Input: dimensioned drawing with shaded views. Units: mm. Origin: part minimum x, y, z. A direction names the side the tool comes from. Round coordinates to 2 decimals unless told otherwise and drop trailing zeros. Loops run counter-clockwise (first coordinate to the right, second up) from the corner with the lowest first, then second, coordinate; pieces in that order, holes last. Notation, with made-up numbers: M -15,22.25 L 42,22.25 A35 ccw 42,54.25 Z; hole C -26,21.5 d4. An arc over 180 degrees is marked long. Use one line per item in the form item = value. Start each with the question number.
Q1. Ray query, line 1 along Z through (x, y) = (12, 0.8); line 2 along X through (y, z) = (3.25, 20); line 3 along Z through (x, y) = (60.8, 21.95). Return the intervals inside material, ascending.
Q2. Section query A-A, the plane x = 60.8. Output: boundary loops of the cut face in (y, z).
Q3. Access query for the marked faces 1, 2 and 3. Directions: +Z, -Z, +X, -X, +Y, -Y. A direction counts if a zero-diameter tool reaches every point of the face in a straight line with its end or side. Return the directions, or none.
Q4. First-contact query: P1, Ø4, axis at x = 12, z = 37.5, coming from the -Y side; P2, Ø2, axis at y = 8.5, z = 15.5, coming from the -X side; P3, Ø5, axis at x = 12, z = 17.5, coming from the +Y side; P4, Ø16, axis at x = 60.8, z = 27.5, coming from the -Y side. Flat tips, straight axial feed; report the tip coordinate or a pass-through.
Q5. Section query C-C, the plane x = 12. Output: boundary loops of the cut face in (y, z).
Q6. Section query D-D, the plane z = 37.5. Output: boundary loops of the cut face in (x, y), and give its area (3 significant figures).
Q7. Section query B-B, the plane z = 27.5. Output: boundary loops of the cut face in (x, y), and give its area (3 significant figures).
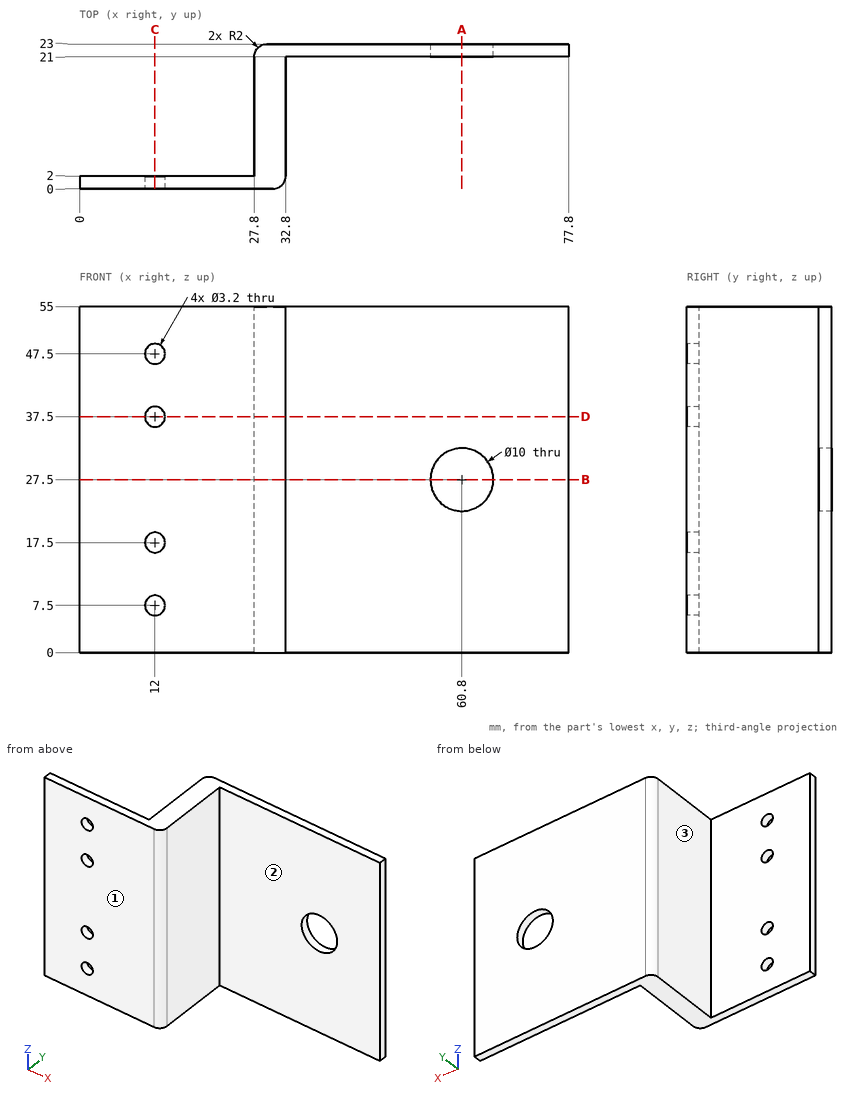
Results found:
q1.line_1 = 0 to 5.9, 9.1 to 15.9, 19.1 to 35.9, 39.1 to 45.9, 49.1 to 55
q1.line_2 = 27.8 to 32.8
q1.line_3 = 0 to 22.5, 32.5 to 55
q2.outline = M 21,0 L 23,0 L 23,22.5 L 21,22.5 Z; M 21,32.5 L 23,32.5 L 23,55 L 21,55 Z
q3.face_1 = +Z, -Z, +X, -X, -Y
q3.face_2 = +Z, -Z, +X, -Y
q3.face_3 = +Z, -Z, -X, +Y
q4.P1 = 0
q4.P2 = 27.8
q4.P3 = 2
q4.P4 = 21
q5.outline = M 0,0 L 2,0 L 2,5.9 L 0,5.9 Z; M 0,9.1 L 2,9.1 L 2,15.9 L 0,15.9 Z; M 0,19.1 L 2,19.1 L 2,35.9 L 0,35.9 Z; M 0,39.1 L 2,39.1 L 2,45.9 L 0,45.9 Z; M 0,49.1 L 2,49.1 L 2,55 L 0,55 Z
q6.outline = M 0,0 L 10.4,0 L 10.4,2 L 0,2 Z; M 13.6,0 L 30.8,0 A2 ccw 32.8,2 L 32.8,21 L 77.8,21 L 77.8,23 L 29.8,23 A2 ccw 27.8,21 L 27.8,2 L 13.6,2 Z
q6.area = 252 mm²
q7.outline = M 0,0 L 30.8,0 A2 ccw 32.8,2 L 32.8,21 L 55.8,21 L 55.8,23 L 29.8,23 A2 ccw 27.8,21 L 27.8,2 L 0,2 Z; M 65.8,21 L 77.8,21 L 77.8,23 L 65.8,23 Z
q7.area = 239 mm²
